```python
from build123d import *

# Parameters (mm, degrees)
BOSS_EXTRUDE1_DEPTH                           = 15.875
BOSS_EXTRUDE2_DEPTH                           = 15.875
CBORE_FOR_1_4_SOCKET_HEAD_CAP_SCREW1_AT_COUNT = 2
CBORE_FOR_1_4_SOCKET_HEAD_CAP_SCREW1_AT_PITCH = 41.275
MOVE_FACE1_BY                                 = 0.127
MOVE_FACE1_2_BY                               = 0.127
MOVE_START                                    = 28.575
MOVE_FACE2_OUTLINE_W                          = 15.875
MOVE_FACE2_OUTLINE_H                          = 60.325
MOVE_FACE2_OUTLINE_R                          = 5.55625
MOVE_FACE2_DEPTH                              = 6.35
MOVE_START_2                                  = 22.225
MOVE_FACE2_2_OUTLINE_R                        = 5.55625
MOVE_FACE2_2_OUTLINE_R_2                      = 3.57124
MOVE_FACE2_2_DEPTH                            = 6.35


with BuildPart() as part:
    # Sketch1 → Boss-Extrude1 (new body)
    with BuildSketch(Plane(origin=(0, 0, 0), x_dir=(0, 0, -1), z_dir=(1, 0, 0))):
        with BuildLine():
            Line((30.1625, 0), (14.2875, 0))
            ThreePointArc((14.2875, 0), (0, -14.2875), (-14.2875, 0))
            Line((-14.2875, 0), (-30.1625, 0))
            Line((-30.1625, 0), (-30.1625, -34.925))
            Line((-30.1625, -34.925), (30.1625, -34.925))
            Line((30.1625, -34.925), (30.1625, 0))
        make_face()
    extrude(amount=BOSS_EXTRUDE1_DEPTH)


with BuildPart() as body_2:
    # Sketch1<3> → Boss-Extrude2 (new body)
    with BuildSketch(Plane(origin=(0, 0, 0), x_dir=(0, 0, -1), z_dir=(1, 0, 0))):
        with BuildLine():
            ThreePointArc((-14.2875, 0), (0, 14.2875), (14.2875, 0))
            Line((14.2875, 0), (30.1625, 0))
            Line((30.1625, 0), (30.1625, 34.925))
            Line((30.1625, 34.925), (-30.1625, 34.925))
            Line((-30.1625, 34.925), (-30.1625, 0))
            Line((-30.1625, 0), (-14.2875, 0))
        make_face()
    extrude(amount=BOSS_EXTRUDE2_DEPTH)


with BuildPart() as cbore_for_1_4_socket_head_cap_screw1_tool:
    # Sketch4 → CBORE for 1/4 Socket Head Cap Screw1 (revolve)
    with BuildSketch(Plane(origin=(7.9375, 34.925, 20.6375), x_dir=(0, 0, 1), z_dir=(1, 0, 0))):
        Polygon((0, 0), (0, 69.85), (3.57124, 69.85), (3.57124, 6.35), (5.55625, 6.35), (5.55625, 0.635), (6.19125, 0), align=None)
    cbore_for_1_4_socket_head_cap_screw1 = revolve(axis=Axis((7.9375, 41.275, 20.6375), (0, -1, 0)))


with BuildPart() as part_1:
    add(part.part)

    # CBORE for 1/4 Socket Head Cap Screw1: cut by cbore_for_1_4_socket_head_cap_screw1_tool
    add(cbore_for_1_4_socket_head_cap_screw1_tool.part, mode=Mode.SUBTRACT)


with BuildPart() as body_2_1:
    add(body_2.part)

    # CBORE for 1/4 Socket Head Cap Screw1: cut by cbore_for_1_4_socket_head_cap_screw1_tool
    add(cbore_for_1_4_socket_head_cap_screw1_tool.part, mode=Mode.SUBTRACT)


with BuildPart() as cbore_for_1_4_socket_head_cap_screw1_at_tool:
    # CBORE for 1/4 Socket Head Cap Screw1 at: CBORE for 1/4 Socket Head Cap Screw1 ×2
    with Locations(*[(0, 0, -i * CBORE_FOR_1_4_SOCKET_HEAD_CAP_SCREW1_AT_PITCH) for i in range(1, CBORE_FOR_1_4_SOCKET_HEAD_CAP_SCREW1_AT_COUNT)]):
        add(cbore_for_1_4_socket_head_cap_screw1)


with BuildPart() as part_2:
    add(part_1.part)

    # CBORE for 1/4 Socket Head Cap Screw1 at: cut by cbore_for_1_4_socket_head_cap_screw1_at_tool
    add(cbore_for_1_4_socket_head_cap_screw1_at_tool.part, mode=Mode.SUBTRACT)

    # Move Face1 2: a curved face moved inward by 0.127
    add(Solid.thicken(part_2.faces().sort_by_distance((7.9375, -14.2875, 0))[0], -MOVE_FACE1_2_BY), mode=Mode.SUBTRACT)

    # Chamfer2
    # the kernel refuses this chamfer: 0.635 mm, written as the material it takes off along each edge
    with BuildSketch(Plane(origin=(0, 0, 0), x_dir=(0, 0.1132288377802066, -0.9935689358544497), z_dir=(0, 0.9935689358544497, 0.1132288377802066))) as chamfer2_piece_1:
        with BuildLine():
            Line((15.067460512, 0.017960512), (14.396539488, -0.652960512))
            Line((14.396539488, -0.652960512), (14.383839488, -0.652960512))
            ThreePointArc((14.383839488, -0.652960512), (14.4018, -0.326480256), (14.4018, 0))
            Line((14.4018, 0), (14.4145, 0.0127))
            ThreePointArc((14.4145, 0.0127), (14.740980256, 0.0127), (15.067460512, 0.030660512))
            Line((15.067460512, 0.030660512), (15.067460512, 0.017960512))
        make_face()
    revolve(axis=Axis((0, 0, 0), (-1, 0, 0)), revolution_arc=193.002955297, mode=Mode.SUBTRACT)
    with BuildSketch(Plane(origin=(-1.600435701, 0, -14.4145), x_dir=(0, 0, -1), z_dir=(1, 0, 0))) as chamfer2_piece_2:
        with BuildLine():
            Line((0.639932919, 0.017577515), (-0.031172593, -0.625784266))
            Line((-0.031172593, -0.625784266), (-0.043861283, -0.625248401))
            ThreePointArc((-0.043861283, -0.625248401), (-0.016099091, -0.31288099), (-0.0127, 0))
            Line((-0.0127, 0), (0, 0.0127))
            ThreePointArc((0, 0.0127), (0.319966459, 0.0127), (0.639932919, 0.030277515))
            Line((0.639932919, 0.030277515), (0.639932919, 0.017577515))
        make_face()
    extrude(amount=19.075871403, mode=Mode.SUBTRACT)
    with BuildSketch(Plane(origin=(-1.600435701, 0, 14.4145), x_dir=(0, -0.999777333387341, -0.021101745067597762), z_dir=(1, 0, 0))) as chamfer2_piece_3:
        with BuildLine():
            Line((0.626302721, 0.017960512), (-0.031077302, -0.639419511))
            Line((-0.031077302, -0.639419511), (-0.043774474, -0.639151519))
            ThreePointArc((-0.043774474, -0.639151519), (-0.019449023, -0.319627221), (-0.012697172, 0.000267992))
            Line((-0.012697172, 0.000267992), (0.000267992, 0.012697172))
            ThreePointArc((0.000267992, 0.012697172), (0.313151041, 0.009493172), (0.626034729, 0.030657684))
            Line((0.626034729, 0.030657684), (0.626302721, 0.017960512))
        make_face()
    extrude(amount=19.075871403, mode=Mode.SUBTRACT)
    with BuildSketch(Plane(origin=(15.875, 0, 0), x_dir=(0, 0.11322883778020662, -0.9935689358544497), z_dir=(0, 0.9935689358544497, 0.11322883778020662))) as chamfer2_piece_4:
        with BuildLine():
            Line((14.396539488, 0.652960512), (15.067460512, -0.017960512))
            Line((15.067460512, -0.017960512), (15.067460512, -0.030660512))
            ThreePointArc((15.067460512, -0.030660512), (14.740980256, -0.0127), (14.4145, -0.0127))
            Line((14.4145, -0.0127), (14.4018, 0))
            ThreePointArc((14.4018, 0), (14.4018, 0.326480256), (14.383839488, 0.652960512))
            Line((14.383839488, 0.652960512), (14.396539488, 0.652960512))
        make_face()
    revolve(axis=Axis((15.875, 0, 0), (-1, 0, 0)), revolution_arc=193.002955297, mode=Mode.SUBTRACT)


with BuildPart() as body_2_2:
    add(body_2_1.part)

    # CBORE for 1/4 Socket Head Cap Screw1 at: cut by cbore_for_1_4_socket_head_cap_screw1_at_tool
    add(cbore_for_1_4_socket_head_cap_screw1_at_tool.part, mode=Mode.SUBTRACT)

    # Move Face1: a curved face moved inward by 0.127
    add(Solid.thicken(body_2_2.faces().sort_by_distance((7.9375, 14.2875, 0))[0], -MOVE_FACE1_BY), mode=Mode.SUBTRACT)

    # Move Face2: read off the stored shape, not the designer's step
    # Move Face2 outline → Move Face2 (cut)
    with BuildSketch(Plane(origin=(0, 0, 0), x_dir=(1, 0, 0), z_dir=(0, 1, 0)).offset(MOVE_START)):
        with Locations((7.9375, 0)):
            Rectangle(MOVE_FACE2_OUTLINE_W, MOVE_FACE2_OUTLINE_H)
        with Locations((7.9375, -20.6375)):
            Circle(MOVE_FACE2_OUTLINE_R, mode=Mode.SUBTRACT)
        with Locations((7.9375, 20.6375)):
            Circle(MOVE_FACE2_OUTLINE_R, mode=Mode.SUBTRACT)
    extrude(amount=MOVE_FACE2_DEPTH, mode=Mode.SUBTRACT)

    # Move Face2 2 outline → Move Face2 2 (cut)
    # profile 1 of 2: a face of its own
    with BuildSketch(Plane(origin=(0, 0, 0), x_dir=(1, 0, 0), z_dir=(0, 1, 0)).offset(MOVE_START_2)):
        with Locations((7.9375, 20.6375)):
            Circle(MOVE_FACE2_2_OUTLINE_R)
        with Locations((7.9375, 20.6375)):
            Circle(MOVE_FACE2_2_OUTLINE_R_2, mode=Mode.SUBTRACT)
    # profile 2 of 2: a face of its own
    with BuildSketch(Plane(origin=(0, 0, 0), x_dir=(1, 0, 0), z_dir=(0, 1, 0)).offset(MOVE_START_2)):
        with Locations((7.9375, -20.6375)):
            Circle(MOVE_FACE2_2_OUTLINE_R)
        with Locations((7.9375, -20.6375)):
            Circle(MOVE_FACE2_2_OUTLINE_R_2, mode=Mode.SUBTRACT)
    extrude(amount=MOVE_FACE2_2_DEPTH, mode=Mode.SUBTRACT)

    # Move Face2 3: loft between two sections, ruled curve by curve
    move_face2_3_from = [
        Edge.make_three_point_arc((7.9375, 27.94, -15.08125), (13.49375, 27.94, -20.6375), (7.9375, 27.94, -26.19375)),
        Edge.make_three_point_arc((7.9375, 27.94, -26.19375), (2.38125, 27.94, -20.6375), (7.9375, 27.94, -15.08125)),
    ]
    move_face2_3_to = [
        Edge.make_three_point_arc((7.9375, 28.575, -14.44625), (14.12875, 28.575, -20.6375), (7.9375, 28.575, -26.82875)),
        Edge.make_three_point_arc((7.9375, 28.575, -26.82875), (1.74625, 28.575, -20.6375), (7.9375, 28.575, -14.44625)),
    ]
    move_face2_3 = Solid(Shell([*[Face.make_surface_from_curves(move_face2_3_from[k], move_face2_3_to[k]) for k in range(2)], Face(Wire(move_face2_3_from)), Face(Wire(move_face2_3_to))]))
    add(move_face2_3, mode=Mode.SUBTRACT)

    # Move Face2 4: loft between two sections, ruled curve by curve
    move_face2_4_from = [
        Edge.make_three_point_arc((7.9375, 27.94, 26.19375), (13.49375, 27.94, 20.6375), (7.9375, 27.94, 15.08125)),
        Edge.make_three_point_arc((7.9375, 27.94, 15.08125), (2.38125, 27.94, 20.6375), (7.9375, 27.94, 26.19375)),
    ]
    move_face2_4_to = [
        Edge.make_three_point_arc((7.9375, 28.575, 26.82875), (14.12875, 28.575, 20.6375), (7.9375, 28.575, 14.44625)),
        Edge.make_three_point_arc((7.9375, 28.575, 14.44625), (1.74625, 28.575, 20.6375), (7.9375, 28.575, 26.82875)),
    ]
    move_face2_4 = Solid(Shell([*[Face.make_surface_from_curves(move_face2_4_from[k], move_face2_4_to[k]) for k in range(2)], Face(Wire(move_face2_4_from)), Face(Wire(move_face2_4_to))]))
    add(move_face2_4, mode=Mode.SUBTRACT)

    # Chamfer1
    # the kernel refuses this chamfer: 0.635 mm, written as the material it takes off along each edge
    with BuildSketch(Plane(origin=(0, 0, 0), x_dir=(0, -0.11322883778020673, 0.9935689358544497), z_dir=(0, -0.9935689358544497, -0.11322883778020673))) as chamfer1_piece_1:
        with BuildLine():
            Line((15.067460512, 0.017960512), (14.396539488, -0.652960512))
            Line((14.396539488, -0.652960512), (14.383839488, -0.652960512))
            ThreePointArc((14.383839488, -0.652960512), (14.4018, -0.326480256), (14.4018, 0))
            Line((14.4018, 0), (14.4145, 0.0127))
            ThreePointArc((14.4145, 0.0127), (14.740980256, 0.0127), (15.067460512, 0.030660512))
            Line((15.067460512, 0.030660512), (15.067460512, 0.017960512))
        make_face()
    revolve(axis=Axis((0, 0, 0), (-1, 0, 0)), revolution_arc=193.002955297, mode=Mode.SUBTRACT)
    with BuildSketch(Plane(origin=(-1.600435701, 0, 14.4145), x_dir=(0, 0, 1), z_dir=(1, 0, 0))) as chamfer1_piece_2:
        with BuildLine():
            Line((0.639932919, 0.017577515), (-0.031172593, -0.625784266))
            Line((-0.031172593, -0.625784266), (-0.043861283, -0.625248401))
            ThreePointArc((-0.043861283, -0.625248401), (-0.016099091, -0.31288099), (-0.0127, 0))
            Line((-0.0127, 0), (0, 0.0127))
            ThreePointArc((0, 0.0127), (0.319966459, 0.0127), (0.639932919, 0.030277515))
            Line((0.639932919, 0.030277515), (0.639932919, 0.017577515))
        make_face()
    extrude(amount=19.075871403, mode=Mode.SUBTRACT)
    with BuildSketch(Plane(origin=(-1.600435701, 0, -14.4145), x_dir=(0, 0.999777333387341, 0.021101745067597762), z_dir=(1, 0, 0))) as chamfer1_piece_3:
        with BuildLine():
            Line((0.626302721, 0.017960512), (-0.031077302, -0.639419511))
            Line((-0.031077302, -0.639419511), (-0.043774474, -0.639151519))
            ThreePointArc((-0.043774474, -0.639151519), (-0.019449023, -0.319627221), (-0.012697172, 0.000267992))
            Line((-0.012697172, 0.000267992), (0.000267992, 0.012697172))
            ThreePointArc((0.000267992, 0.012697172), (0.313151041, 0.009493172), (0.626034729, 0.030657684))
            Line((0.626034729, 0.030657684), (0.626302721, 0.017960512))
        make_face()
    extrude(amount=19.075871403, mode=Mode.SUBTRACT)
    with BuildSketch(Plane(origin=(15.875, 0, 0), x_dir=(0, -0.11322883778020675, 0.9935689358544497), z_dir=(0, -0.9935689358544497, -0.11322883778020675))) as chamfer1_piece_4:
        with BuildLine():
            Line((14.396539488, 0.652960512), (15.067460512, -0.017960512))
            Line((15.067460512, -0.017960512), (15.067460512, -0.030660512))
            ThreePointArc((15.067460512, -0.030660512), (14.740980256, -0.0127), (14.4145, -0.0127))
            Line((14.4145, -0.0127), (14.4018, 0))
            ThreePointArc((14.4018, 0), (14.4018, 0.326480256), (14.383839488, 0.652960512))
            Line((14.383839488, 0.652960512), (14.396539488, 0.652960512))
        make_face()
    revolve(axis=Axis((15.875, 0, 0), (-1, 0, 0)), revolution_arc=193.002955297, mode=Mode.SUBTRACT)


solid = part_2.part
```
Here's how the part is built. I have some questions about the finished solid (model axes, mm). Give positions to 0.01 mm unless a question says otherwise; leave off trailing zeros. Write each loop counter-clockwise with the first axis right and the second up, starting at its lowest first coordinate (ties: lowest second). Pieces come first, ordered by that corner, then holes. Notation, with made-up numbers: M 59,13 L 65,13 A28 ccw 65,48 Z; hole C -17,3.25 d7. An arc over 180 degrees is marked long. Put each result on its own line as item: value. Start each with the question number.
Item 1: If we section it at C-C, the plane z = 0: Write out the boundary of the cut face in (x, y) (1 decimal).
Item 2: Thinking about a two-plate mould opening in Z: for faces 1 (the conical face through (0.463, -14.583, -0.321)), 2 (the flat face through (15.875, -21, 0)), 3 (the cylindrical face through (5.524, -17.218, -23.27)), 4 (the flat face through (8, -18, -30.162)), which applies, +Z half, -Z half, draft (parallel to the pull), parting line (faces both ways), or undercut?
Item 3: Will this pin go through, and if not, where does the flat tip stop? pin 1 (8 mm diameter, centred on y = -18, z = -19, fed in from -X).
Item 4: If we section it at D-D, the plane x = 9.75: Write out the boundary of the cut face in (y, z) (1 decimal), then the cut area to 3 significant figures.
Item 5: I need wall thicknesses on L1, parallel to Z at x = 8.25, y = -16; L2, parallel to Z at x = 6.5, y = -17.5; L3, parallel to Z at x = 6, y = -7. Which ranges of each line are inside material? Lowest first, please. Write a range as from..to.
Item 6: If we section it at B-B, the plane x = 2.5: Write out the boundary of the cut face in (y, z) (1 decimal).
Item 7: If we section it at A-A, the plane z = -18: Write out the boundary of the cut face in (x, y) (3 decimals).
Values:
1. outline: M 0,-34.9 L 15.9,-34.9 L 15.9,-15 L 15.2,-14.4 L 0.6,-14.4 L 0,-15 Z
2. face 1: undercut
2. face 2: draft
2. face 3: undercut
2. face 4: -Z half
3. pin 1: x = 0
4. outline: M -34.9,-30.2 L 0,-30.2 L 0,-23.7 L -34.9,-23.7 Z; M -34.9,-17.6 L 0,-17.6 L 0,-15 L -0.6,-14.4 A14.4 cw -0.6,14.4 L 0,15 L 0,17.6 L -34.9,17.6 Z; M -34.9,23.7 L 0,23.7 L 0,30.2 L -34.9,30.2 Z
4. area: 1,350 mm²
5. L1: -30.16..-24.2, -17.08..17.08, 24.2..30.16
5. L2: -30.16..-23.91, -17.37..17.37, 23.91..30.16
5. L3: -30.16..-23.64, -17.64..-12.6, 12.6..17.64, 23.64..30.16
6. outline: M -34.9,-30.2 L 0,-30.2 L 0,-15 L -0.6,-14.4 A14.4 cw -0.6,14.4 L 0,15 L 0,30.2 L -34.9,30.2 Z
7. outline: M 0,-34.925 L 5.53,-34.925 L 5.53,0 L 0,0 Z; M 10.345,-34.925 L 15.875,-34.925 L 15.875,0 L 10.345,0 Z
